Print and shaded views of the part. All mm, measured from the part's lowest x, y and z. A direction names the side the tool comes from. Coordinates: 2 decimals unless noted, no trailing zeros. Order: outer loops, then holes, each group sorted by start corner. A loop starts at its lowest first (then second) coordinate and runs counter-clockwise, first axis right, second up. Notation, with made-up numbers: M -7,-10.75 L 24,-10.75 A25 cw 24,21.25 Z; hole C 4,27 d8. An arc over 180 degrees is marked long. One line per item, written item: value.
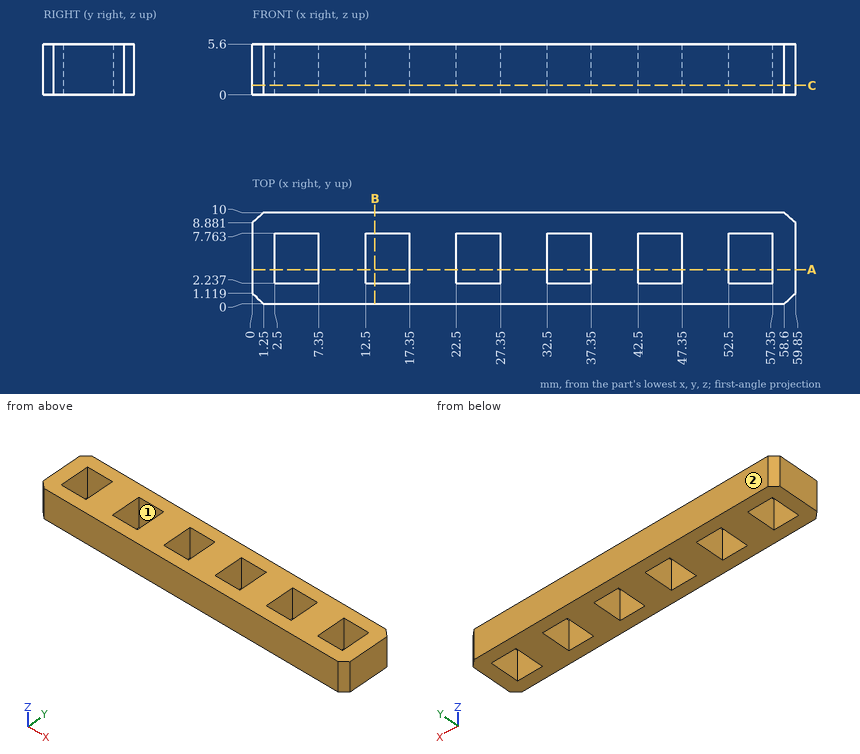
Q1. Slice it at A-A (y = 3.75). List the corners of the cut face in (x, z), plus the area to 3 significant figures.
Recorded:
outline: M 0,0 L 2.5,0 L 2.5,5.6 L 0,5.6 Z; M 7.35,0 L 12.5,0 L 12.5,5.6 L 7.35,5.6 Z; M 17.35,0 L 22.5,0 L 22.5,5.6 L 17.35,5.6 Z; M 27.35,0 L 32.5,0 L 32.5,5.6 L 27.35,5.6 Z; M 37.35,0 L 42.5,0 L 42.5,5.6 L 37.35,5.6 Z; M 47.35,0 L 52.5,0 L 52.5,5.6 L 47.35,5.6 Z; M 57.35,0 L 59.85,0 L 59.85,5.6 L 57.35,5.6 Z
area: 172 mm^2
Q2. Drill centre line: line 1 along Y through (x, z) = (45, 3.25). Where is it in solid material? Low to high.
Recorded:
line 1: y = 0 to 2.24, 7.76 to 10
Q3. Slice it at B-B (x = 13.5). List the corners of the cut face in (y, z).
Recorded:
outline: M 0,0 L 2.24,0 L 2.24,5.6 L 0,5.6 Z; M 7.76,0 L 10,0 L 10,5.6 L 7.76,5.6 Z
Q4. Which spindle directions (+Z, -Z, +X, -X, +Y, -Y) get a long thin tool onto all of the face, cutting with end or side? Do the marked faces 1 and 2. Say none if no direction does.
Recorded:
face 1: +Z, -Z
face 2: +Z, -Z, +X, -X, +Y
Q5. Slice it at C-C (z = 1.05). Give the number of separate pieces and of enclosed holes in the cut face, plus the area to 3 significant figures.
Recorded:
separate pieces: 1
enclosed holes: 6
area: 435 mm^2
